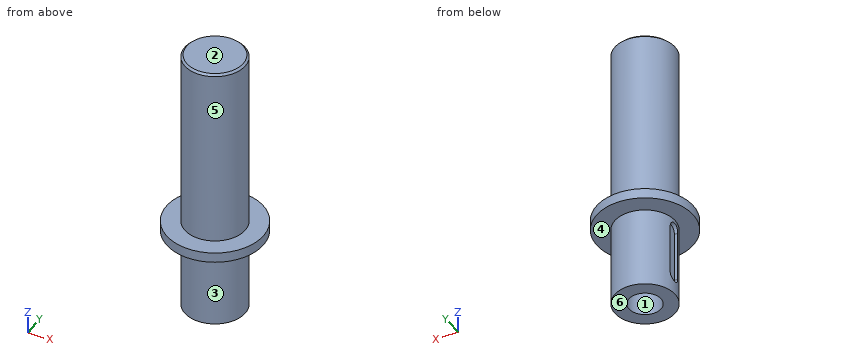
```python
from build123d import *

# Parameters (mm, degrees)
SKETCH1_R           = 15
BOSS_EXTRUDE1_DEPTH = 90
SKETCH2_R           = 24
BOSS_EXTRUDE2_DEPTH = 5
CHAMFER1_SIZE       = 1
BOSS_EXTRUDE3_START = 40
SKETCH4_R           = 15
BOSS_EXTRUDE3_DEPTH = 40
CUT_EXTRUDE1_DEPTH  = 2
SKETCH6_R           = 8
CUT_EXTRUDE2_DEPTH  = 45


with BuildPart() as part:
    # Sketch1 → Boss-Extrude1 (new body)
    with BuildSketch(Plane.XY):
        with Locations(Location((0, 0, 0), (0, 0, 180))):
            Circle(SKETCH1_R)
    extrude(amount=BOSS_EXTRUDE1_DEPTH)

    # Sketch2 → Boss-Extrude2 (add)
    with BuildSketch(Plane(origin=(0, 0, 0), x_dir=(-1, 0, 0), z_dir=(0, 0, -1))):
        Circle(SKETCH2_R)
    extrude(amount=BOSS_EXTRUDE2_DEPTH)

    # Chamfer1
    chamfer1_edges = [part.edges().sort_by_distance(p)[0] for p in [
        (15, 0, 90),
    ]]
    chamfer(chamfer1_edges, length=CHAMFER1_SIZE)

    # Sketch4 → Boss-Extrude3 (add)
    with BuildSketch(Plane(origin=(0, 0, -5), x_dir=(-1, 0, 0), z_dir=(0, 0, -1)).offset(BOSS_EXTRUDE3_START)):
        Circle(SKETCH4_R)
    extrude(amount=-BOSS_EXTRUDE3_DEPTH)

    # Sketch5 → Cut-Extrude1 (cut)
    with BuildSketch(Plane(origin=(-15, 0, -45), x_dir=(0, 0, -1), z_dir=(1, 0, 0))):
        with BuildLine():
            Line((-35, 3.284094305), (-10, 3.284094305))
            ThreePointArc((-10, 3.284094305), (-6.715905695, 0), (-10, -3.284094305))
            Line((-10, -3.284094305), (-35, -3.284094305))
            ThreePointArc((-35, -3.284094305), (-38.284094305, 0), (-35, 3.284094305))
        make_face()
    extrude(amount=CUT_EXTRUDE1_DEPTH, mode=Mode.SUBTRACT)

    # Sketch6 → Cut-Extrude2 (cut)
    with BuildSketch(Plane(origin=(0, 0, -45), x_dir=(-1, 0, 0), z_dir=(0, 0, -1))):
        Circle(SKETCH6_R)
    extrude(amount=-CUT_EXTRUDE2_DEPTH, mode=Mode.SUBTRACT)


solid = part.part
```
Check sheet for the modelled part. Datum: model origin and axes. Units: mm. Face numbers are marked on the shaded views. A direction names the side the tool comes from. Round coordinates to 2 decimals unless told otherwise and drop trailing zeros. Order: outer loops, then holes, each group sorted by start corner. A loop starts at its lowest first (then second) coordinate and runs counter-clockwise, first axis right, second up.
1) Section check A-A (z = -14). Record the boundary of the cut face in (x, y).
2) Section check D-D (z = 45). Record the boundary of the cut face in (x, y).
3) Section check B-B (x = 0). Record the boundary of the cut face in (y, z), and give its area (3 significant figures).
4) Go/stop test with flat-tipped pins: pin 1 Ø7 at (y, z) = (-0.5, -22) entering from -X; pin 2 Ø4 at (x, y) = (14, 5.5) entering from -Z; pin 3 Ø6 at (y, z) = (-10.5, -22) entering from -X; pin 4 Ø12 at (x, z) = (12, -18) entering from -Y. Record where each tip stops, or that it passes through.
5) Section check C-C (y = 0). Record the boundary of the cut face in (x, z), and give its area (3 significant figures).
6) Mould release check, pull along X, two halves, no side actions. Record for the marked faces 1, 2 and 3: +X half, -X half, draft (parallel to the pull), parting line (faces both ways), or undercut.
7) Scan lines: line 1 (Y direction, x = 0, z = -19); line 2 (Z direction, x = 3, y = -5.5); line 3 (Z direction, x = -19, y = 0.5). Record each from-to range of solid material in increasing order.
8) Tool access check on the marked faces 4, 5 and 6. Record the directions out of +Z, -Z, +X, -X, +Y, -Y that give a thin tool (end or side, any length) a straight path to the whole face; none if there is none.
Result:
1. outline: (-14.64, -3.28) arc R15 ccw (long way) to (-14.64, 3.28) - (-13, 3.28) - (-13, -3.28) - close; hole circle Ø16 at (0, 0)
2. outline: circle Ø30 at (0, 0)
3. outline: (-24, -5) - (-15, -5) - (-15, -45) - (-8, -45) - (-8, 0) - (8, 0) - (8, -45) - (15, -45) - (15, -5) - (24, -5) - (24, 0) - (15, 0) - (15, 89) - (14, 90) - (-14, 90) - (-15, 89) - (-15, 0) - (-24, 0) - close
3. area: 3,420 mm2
4. pin 1: stops at x = -14.64
4. pin 2: stops at z = -45
4. pin 3: stops at x = -12.99
4. pin 4: stops at y = -13.75
5. outline: (-24, -5) - (-15, -5) - (-15, -6.72) - (-13, -6.72) - (-13, -38.28) - (-15, -38.28) - (-15, -45) - (-8, -45) - (-8, 0) - (8, 0) - (8, -45) - (15, -45) - (15, -5) - (24, -5) - (24, 0) - (15, 0) - (15, 89) - (14, 90) - (-14, 90) - (-15, 89) - (-15, 0) - (-24, 0) - close
5. area: 3,360 mm2
6. face 1: undercut
6. face 2: draft
6. face 3: parting line
7. line 1: y = -15 to -8, 8 to 15
7. line 2: z = 0 to 90
7. line 3: z = -5 to 0
8. face 4: -Z
8. face 5: +Z
8. face 6: -Z, +X, -X, +Y, -Y
